Design review of the part built by this model. Coordinates are the model's own, in mm. A direction names the side the tool comes from. Round coordinates to 2 decimals unless told otherwise and drop trailing zeros. Loops run counter-clockwise (first coordinate to the right, second up) from the corner with the lowest first, then second, coordinate; pieces in that order, holes last. Notation, with made-up numbers: (-19, 43.25) - (33, 43.25) arc R16 cw to (33, 55.25) - close; hole circle Ø5 at (49, 53). An arc over 180 degrees is marked (long way). Return JSON: item names as keys, results as strings. Group by question number.
(1) Clearance check with flat-ended pins moving along their axes: pin 1 (21 mm diameter, centred on x = -31.5, y = 14, fed in from +Z); pin 2 (0.5 mm diameter, centred on x = -43, y = 32, fed in from +Z). State where each tip first meets the part, or that it passes through.
(2) For faces 4 (the flat face through (10, 28, 20)), 5 (the flat face through (-49, 16, 20)), list the 3-axis set-ups (+Z, -Z, +X, -X, +Y, -Y) from which the entire face can be reached by the end or side of a thin tool; tool diameter is ignored.
(3) We need section B-B, the plane y = 34. Write out the cut boundary in (x, z), and give its area (3 significant figures).
(4) We need section A-A, the plane z = 2. Write out the cut boundary in (x, y).
(5) We need section C-C, the plane x = -29. Write out the cut boundary in (y, z), and give its area (3 significant figures).
(6) The part is to be moulded in two halves that separate along X. For faces 1 (the flat face through (-19, -5, 20)), 2 (the flat face through (11, 11, 20)), 3 (the flat face through (-19, -6, 20)), say which applies: pulls with the +X half, pulls with the -X half, needs draft (parallel to the pull), parting line crosses it, or undercut.
(7) Wall thickness on L1, parallel to Y at x = -43, z = 4; L2, parallel to X at y = 27.5, z = 13; L3, parallel to Y at x = -44, z = 37.5: over which ranges is each line inside the solid? List them lowest first. Write a range as [from, to].
(8) We need section D-D, the plane z = 22. Write out the cut boundary in (x, y).
from build123d import *

# Parameters (mm, degrees)
F1_DEPTH = 40
F0_W     = 1
F0_H     = 7
F2_DEPTH = 1
F3_DEPTH = 10


with BuildPart() as f1:
    # F0 (on Top) → F1 (new body)
    with BuildSketch(Plane.XY):
        Polygon((10, -5), (-48, -5), (-48, 37), (10, 37), (10, 19.5), (11, 19.5), (11, 38), (-49, 38), (-49, -6), (11, -6), (11, 12.5), (10, 12.5), align=None)
    extrude(amount=F1_DEPTH)

    # F0 (on Top) → F2 (join)
    with BuildSketch(Plane.XY):
        Polygon((-48, 37), (-48, -5), (10, -5), (10, 12.5), (10, 19.5), (10, 37), align=None)
        with BuildLine():
            Line((-0.5, 0), (-42.5, 0))
            ThreePointArc((-42.5, 0), (-43.3535533906, -0.3535533906), (-43, 0.5))
            Line((-43, 0.5), (-43, 31.5))
            ThreePointArc((-43, 31.5), (-43.3535533906, 32.3535533906), (-42.5, 32))
            Line((-42.5, 32), (-0.5, 32))
            ThreePointArc((-0.5, 32), (0, 32.5), (0.5, 32))
            ThreePointArc((0.5, 32), (0.3535533906, 31.6464466094), (0, 31.5))
            Line((0, 31.5), (0, 0.5))
            ThreePointArc((0, 0.5), (0.3535533906, 0.3535533906), (0.5, 0))
            ThreePointArc((0.5, 0), (0, -0.5), (-0.5, 0))
        make_face(mode=Mode.SUBTRACT)
        with BuildLine():
            ThreePointArc((-43, 0.5), (-42.6464466094, 0.3535533906), (-42.5, 0))
            Line((-42.5, 0), (-0.5, 0))
            ThreePointArc((-0.5, 0), (-0.3535533906, 0.3535533906), (0, 0.5))
            Line((0, 0.5), (0, 31.5))
            ThreePointArc((0, 31.5), (-0.3535533906, 31.6464466094), (-0.5, 32))
            Line((-0.5, 32), (-42.5, 32))
            ThreePointArc((-42.5, 32), (-42.6464466094, 31.6464466094), (-43, 31.5))
            Line((-43, 31.5), (-43, 0.5))
        make_face()
        Polygon((10, -5), (-48, -5), (-48, 37), (10, 37), (10, 19.5), (11, 19.5), (11, 38), (-49, 38), (-49, -6), (11, -6), (11, 12.5), (10, 12.5), align=None)
        with Locations((10.5, 16)):
            Rectangle(F0_W, F0_H)
        with BuildLine():
            Line((-42.5, 0), (-43, 0))
            Line((-43, 0), (-43, 0.5))
            ThreePointArc((-43, 0.5), (-43.3535533906, -0.3535533906), (-42.5, 0))
        make_face()
        with BuildLine():
            Line((0, 0), (-0.5, 0))
            ThreePointArc((-0.5, 0), (0, -0.5), (0.5, 0))
            ThreePointArc((0.5, 0), (0.3535533906, 0.3535533906), (0, 0.5))
            Line((0, 0.5), (0, 0))
        make_face()
        with BuildLine():
            Line((0, 32), (0, 31.5))
            ThreePointArc((0, 31.5), (0.3535533906, 31.6464466094), (0.5, 32))
            ThreePointArc((0.5, 32), (0, 32.5), (-0.5, 32))
            Line((-0.5, 32), (0, 32))
        make_face()
        with BuildLine():
            ThreePointArc((-42.5, 32), (-43.3535533906, 32.3535533906), (-43, 31.5))
            Line((-43, 31.5), (-43, 32))
            Line((-43, 32), (-42.5, 32))
        make_face()
        with BuildLine():
            Line((-43, 0.5), (-43, 0))
            Line((-43, 0), (-42.5, 0))
            ThreePointArc((-42.5, 0), (-42.6464466094, 0.3535533906), (-43, 0.5))
        make_face()
        with BuildLine():
            ThreePointArc((0, 0.5), (-0.3535533906, 0.3535533906), (-0.5, 0))
            Line((-0.5, 0), (0, 0))
            Line((0, 0), (0, 0.5))
        make_face()
        with BuildLine():
            ThreePointArc((-0.5, 32), (-0.3535533906, 31.6464466094), (0, 31.5))
            Line((0, 31.5), (0, 32))
            Line((0, 32), (-0.5, 32))
        make_face()
        with BuildLine():
            Line((-43, 32), (-43, 31.5))
            ThreePointArc((-43, 31.5), (-42.6464466094, 31.6464466094), (-42.5, 32))
            Line((-42.5, 32), (-43, 32))
        make_face()
    extrude(amount=F2_DEPTH)

    # F0 (on Top) → F3 (join)
    with BuildSketch(Plane.XY):
        with BuildLine():
            ThreePointArc((-42.5, 32), (-43.3535533906, 32.3535533906), (-43, 31.5))
            Line((-43, 31.5), (-43, 32))
            Line((-43, 32), (-42.5, 32))
        make_face()
        with BuildLine():
            Line((-43, 32), (-43, 31.5))
            ThreePointArc((-43, 31.5), (-42.6464466094, 31.6464466094), (-42.5, 32))
            Line((-42.5, 32), (-43, 32))
        make_face()
        with BuildLine():
            ThreePointArc((-0.5, 32), (-0.3535533906, 31.6464466094), (0, 31.5))
            Line((0, 31.5), (0, 32))
            Line((0, 32), (-0.5, 32))
        make_face()
        with BuildLine():
            Line((0, 32), (0, 31.5))
            ThreePointArc((0, 31.5), (0.3535533906, 31.6464466094), (0.5, 32))
            ThreePointArc((0.5, 32), (0, 32.5), (-0.5, 32))
            Line((-0.5, 32), (0, 32))
        make_face()
        with BuildLine():
            Line((0, 0), (-0.5, 0))
            ThreePointArc((-0.5, 0), (0, -0.5), (0.5, 0))
            ThreePointArc((0.5, 0), (0.3535533906, 0.3535533906), (0, 0.5))
            Line((0, 0.5), (0, 0))
        make_face()
        with BuildLine():
            ThreePointArc((0, 0.5), (-0.3535533906, 0.3535533906), (-0.5, 0))
            Line((-0.5, 0), (0, 0))
            Line((0, 0), (0, 0.5))
        make_face()
        with BuildLine():
            Line((-43, 0.5), (-43, 0))
            Line((-43, 0), (-42.5, 0))
            ThreePointArc((-42.5, 0), (-42.6464466094, 0.3535533906), (-43, 0.5))
        make_face()
        with BuildLine():
            Line((-42.5, 0), (-43, 0))
            Line((-43, 0), (-43, 0.5))
            ThreePointArc((-43, 0.5), (-43.3535533906, -0.3535533906), (-42.5, 0))
        make_face()
    extrude(amount=F3_DEPTH)


solid = f1.part
Solutions:
{
 "1": {"pin 1": "z = 1", "pin 2": "z = 10"},
 "2": {"face 4": "+Z", "face 5": "+Z, -Z, -X, +Y, -Y"},
 "3": {"outline": "(-49, 0) - (11, 0) - (11, 40) - (10, 40) - (10, 1) - (-48, 1) - (-48, 40) - (-49, 40) - close", "area": "138 mm^2"},
 "4": {"outline": "(-49, -6) - (11, -6) - (11, 12.5) - (10, 12.5) - (10, -5) - (-48, -5) - (-48, 37) - (10, 37) - (10, 19.5) - (11, 19.5) - (11, 38) - (-49, 38) - close; circle Ø1 at (-43, 0); circle Ø1 at (-43, 32); circle Ø1 at (0, 0); circle Ø1 at (0, 32)"},
 "5": {"outline": "(-6, 0) - (38, 0) - (38, 40) - (37, 40) - (37, 1) - (-5, 1) - (-5, 40) - (-6, 40) - close", "area": "122 mm^2"},
 "6": {"face 1": "undercut", "face 2": "pulls with the +X half", "face 3": "needs draft"},
 "7": {"L1": "[-6, -5], [-0.5, 0.5], [31.5, 32.5], [37, 38]", "L2": "[-49, -48], [10, 11]", "L3": "[-6, -5], [37, 38]"},
 "8": {"outline": "(-49, -6) - (11, -6) - (11, 12.5) - (10, 12.5) - (10, -5) - (-48, -5) - (-48, 37) - (10, 37) - (10, 19.5) - (11, 19.5) - (11, 38) - (-49, 38) - close"}
}
